Read the model definition and answer for the solid it produces. Units are mm, in the model's axes. Coordinates: 2 decimals unless noted, no trailing zeros. Loops run counter-clockwise (first coordinate to the right, second up) from the corner with the lowest first, then second, coordinate; pieces in that order, holes last. Notation, with made-up numbers: M 77,24.25 L 129,24.25 A20 cw 129,61.25 Z; hole C 86.25,35 d3. An arc over 180 degrees is marked long. Put each result on its own line as item: value.
from build123d import *

# Parameters (mm, degrees)
BOSS_EXTRUDE1_DEPTH = 10
CUT_EXTRUDE6_DEPTH  = 14
SKETCH11_R          = 1.65
CUT_EXTRUDE7_DEPTH  = 3


with BuildPart() as part:
    # Sketch1 → Boss-Extrude1 (new body)
    with BuildSketch(Plane(origin=(0, 0, 0), x_dir=(1, 0, 0), z_dir=(0, 1, 0))):
        Polygon((4.561067127, 0), (2.280533563, 3.95), (-2.280533563, 3.95), (-4.561067127, 0), (-2.280533563, -3.95), (2.280533563, -3.95), align=None)
    extrude(amount=BOSS_EXTRUDE1_DEPTH)

    # Sketch9 → Cut-Extrude6 (cut)
    with BuildSketch(Plane(origin=(0, 10, 0), x_dir=(1, 0, 0), z_dir=(0, 1, 0))):
        with BuildLine():
            Line((-1.217575979, -1.113556795), (1.217575979, -1.113556795))
            ThreePointArc((1.217575979, -1.113556795), (0, 1.65), (-1.217575979, -1.113556795))
        make_face()
    extrude(amount=-CUT_EXTRUDE6_DEPTH, mode=Mode.SUBTRACT)

    # Sketch11 → Cut-Extrude7 (cut)
    with BuildSketch(Plane(origin=(0, 10, 0), x_dir=(1, 0, 0), z_dir=(0, 1, 0))):
        with Locations(Location((0, 0, 0), (0, 0, 317.554942162))):
            Circle(SKETCH11_R)
    extrude(amount=-CUT_EXTRUDE7_DEPTH, mode=Mode.SUBTRACT)


solid = part.part
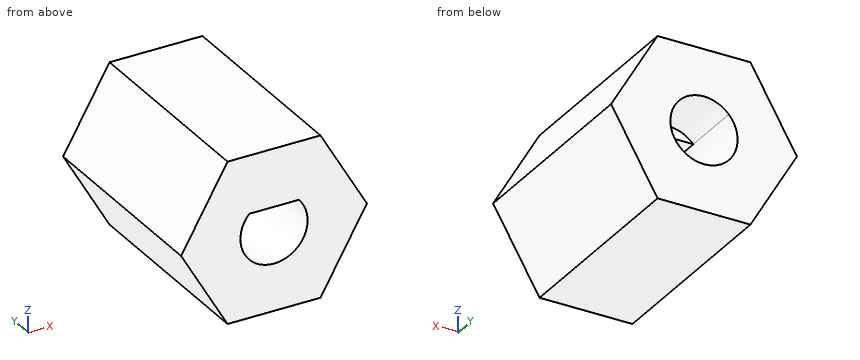
1) Find section C-C, the plane z = -1.5. Write down the section's boundary in (x, y), plus the area to 3 significant figures.
Answer list:
outline: M -3.7,0 L -0.69,0 L -0.69,10 L -3.7,10 Z; M 0.69,0 L 3.7,0 L 3.7,10 L 0.69,10 Z
area: 60.2 mm^2
2) Find section D-D, the plane x = 1. Write down the section's boundary in (y, z), plus the area to 3 significant figures.
Answer list:
outline: M 0,-3.95 L 10,-3.95 L 10,-1.31 L 0,-1.31 Z; M 0,1.11 L 7,1.11 L 7,1.31 L 10,1.31 L 10,3.95 L 0,3.95 Z
area: 54.1 mm^2
3) Find section B-B, the plane y = 8.5. Write down the section's boundary in (x, z), plus the area to 3 significant figures.
Answer list:
outline: M -4.56,0 L -2.28,-3.95 L 2.28,-3.95 L 4.56,0 L 2.28,3.95 L -2.28,3.95 Z; hole C 0,0 d3.3
area: 45.5 mm^2
4) Straight lines are drawn through the part: line 1 (Z direction, x = 0, y = 6.25); line 2 (Z direction, x = 1, y = 4.5); line 3 (Z direction, x = -2.75, y = 9). For each, find the intervals that lie inside material, in ascending order. Write a range as [from, to].
Answer list:
line 1: z = [-3.95, -1.65], [1.11, 3.95]
line 2: z = [-3.95, -1.31], [1.11, 3.95]
line 3: z = [-3.14, 3.14]
5) Find section A-A, the plane x = 0. Write down the section's boundary in (y, z), plus the area to 3 significant figures.
Answer list:
outline: M 0,-3.95 L 10,-3.95 L 10,-1.65 L 0,-1.65 Z; M 0,1.11 L 7,1.11 L 7,1.65 L 10,1.65 L 10,3.95 L 0,3.95 Z
area: 49.8 mm^2
6) Given pin 1 Ø1.5 at (x, y) = (3.5, 2) entering from -Z; pin 2 Ø1.5 at (y, z) = (5.5, 1) entering from +X, each flat-ended and moving along its own axis, determine where each tip first touches the part or whether it passes through.
Answer list:
pin 1: stops at z = -3.14
pin 2: stops at x = 4.42
